from build123d import *

# Parameters (mm, degrees)
F0_W     = 1500
F0_H     = 2500
F1_DEPTH = 1
F2_W     = 2
F2_H     = 2
F2_W_2   = 1496
F2_H_2   = 2496
F3_DEPTH = 7
F4_W     = 7
F4_H     = 7
F4_W_2   = 1486
F4_H_2   = 2486
F5_DEPTH = 2


with BuildPart() as f1:
    # F0 (on Front) → F1 (new body, symmetric)
    with BuildSketch(Plane.XZ):
        with Locations((-750, 1250)):
            Rectangle(F0_W, F0_H)
    extrude(amount=F1_DEPTH, both=True)

    # F2 (on face) → F3 (join)
    with BuildSketch(Plane.XZ.offset(1)):
        with Locations((-1499, 2499)):
            Rectangle(F2_W, F2_H)
        with Locations((-750, 2499)):
            Rectangle(F2_W_2, F2_H)
        with Locations((-1499, 1250)):
            Rectangle(F2_W, F2_H_2)
        with Locations((-1, 2499)):
            Rectangle(F2_W, F2_H)
        with Locations((-1499, 1)):
            Rectangle(F2_W, F2_H)
        with Locations((-750, 1)):
            Rectangle(F2_W_2, F2_H)
        with Locations((-1, 1250)):
            Rectangle(F2_W, F2_H_2)
        with Locations((-1, 1)):
            Rectangle(F2_W, F2_H)
    extrude(amount=F3_DEPTH)

    # F4 (on face) → F5 (join)
    with BuildSketch(Plane.XZ.offset(8)):
        with Locations((-1496.5, 2496.5)):
            Rectangle(F4_W, F4_H)
        with Locations((-750, 2496.5)):
            Rectangle(F4_W_2, F4_H)
        with Locations((-1496.5, 1250)):
            Rectangle(F4_W, F4_H_2)
        with Locations((-3.5, 2496.5)):
            Rectangle(F4_W, F4_H)
        with Locations((-1496.5, 3.5)):
            Rectangle(F4_W, F4_H)
        with Locations((-750, 3.5)):
            Rectangle(F4_W_2, F4_H)
        with Locations((-3.5, 1250)):
            Rectangle(F4_W, F4_H_2)
        with Locations((-3.5, 3.5)):
            Rectangle(F4_W, F4_H)
    extrude(amount=F5_DEPTH)


solid = f1.part
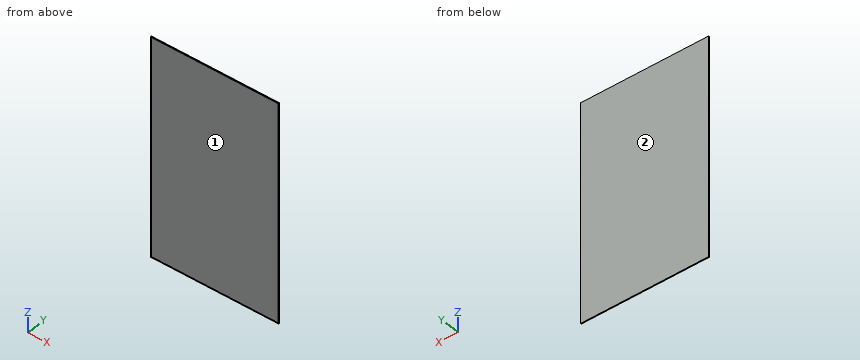
The model under review builds one solid part; all positions refer to its coordinate system, in mm. Face numbers are marked on the shaded views. Round coordinates to 2 decimals unless told otherwise and drop trailing zeros. Write each loop counter-clockwise with the first axis right and the second up, starting at its lowest first coordinate (ties: lowest second). Pieces come first, ordered by that corner, then holes. Notation, with made-up numbers: (-29.5, -25) - (-11.5, -25) arc R27 ccw to (-11.5, -3) - close; hole circle Ø9 at (38.5, 73). An arc over 180 degrees is marked (long way). One line per item, written item: value. Start each with the question number.
1. The part is to be moulded in two halves that separate along Z. For the marked faces 1 and 2, say which applies: released by +Z, released by -Z, zero draft, split by the parting line, or undercut.
2. To check wall thickness, follow L1, parallel to X at y = -6.5, z = 239.5; L2, parallel to Z at x = -846, y = -7.75; L3, parallel to Z at x = -576, y = -8.5. State the ranges of each line that lie inside material, in increasing order. Write a range as from..to.
3. Clearance check with a flat-ended pin moving along its axis: P1, Ø6, axis at x = -446.5, z = 1206.5, coming from the -Y side. State where the tip first meets the part, or that it passes through.
4. Consider section C-C on z = 1150. Write out the cut boundary in (x, y), and give its area (3 significant figures).
5. Consider section B-B on x = -690. Write out the cut boundary in (y, z).
6. Consider section A-A on y = -3.25. Write out the cut boundary in (x, z), and give its area (3 significant figures).
Checks:
1. face 1: undercut
1. face 2: zero draft
2. L1: x = -1500..-1498, -2..0
2. L2: z = 0..2, 2498..2500
2. L3: z = 0..7, 2493..2500
3. P1: stops at y = -1
4. outline: (-1500, -10) - (-1493, -10) - (-1493, -8) - (-1498, -8) - (-1498, -1) - (-2, -1) - (-2, -8) - (-7, -8) - (-7, -10) - (0, -10) - (0, 1) - (-1500, 1) - close
4. area: 3,060 mm^2
5. outline: (-10, 0) - (1, 0) - (1, 2500) - (-10, 2500) - (-10, 2493) - (-8, 2493) - (-8, 2498) - (-1, 2498) - (-1, 2) - (-8, 2) - (-8, 7) - (-10, 7) - close
6. outline: (-1500, 0) - (0, 0) - (0, 2500) - (-1500, 2500) - close; hole (-1498, 2) - (-2, 2) - (-2, 2498) - (-1498, 2498) - close
6. area: 16,000 mm^2
